Geometry: final body of the model. Coordinates: model frame, mm. Face numbers are marked on the shaded views. A direction names the side the tool comes from. Give positions to 0.01 mm unless a question says otherwise; leave off trailing zeros. Write each loop counter-clockwise with the first axis right and the second up, starting at its lowest first coordinate (ties: lowest second). Pieces come first, ordered by that corner, then holes. Notation, with made-up numbers: (-31.75, 80) -> (-19.75, 80) arc R18 cw to (-19.75, 94) -> close; hole circle Ø9 at (47.25, 84). An arc over 180 degrees is marked (long way). Answer in a Markdown table with one row per item. Add a question column.
Item 1: First-contact query: P1, Ø6.5, axis at x = 0, z = 0, coming from the -Y side; P2, Ø1.5, axis at y = 2.5, z = -1.5, coming from the +X side; P3, Ø2, axis at x = 4.5, y = 1.5, coming from the +Z side. Flat tips, straight axial feed; report the tip coordinate or a pass-through.
Item 2: Material intervals for probe 1 along Z at (x, y) = (0, 0.1); probe 2 along Z at (x, y) = (0, 3.95); probe 3 along X at (y, z) = (3.9, 0), sorted ascending. Write a range as from..to.
Item 3: Access query for the marked faces 1 and 2. Directions: +Z, -Z, +X, -X, +Y, -Y. A direction counts if a zero-diameter tool reaches every point of the face in a straight line with its end or side. Return the directions, or none.
Item 4: Section query C-C on y = 1.4. Output: boundary loops of the cut face in (x, z), plus the area to 3 significant figures.
Item 5: Draft query along Z for the marked faces 3, 4 and 5. Return one class per face: +Z half, -Z half, draft (parallel to the pull), parting line (faces both ways), or undercut.
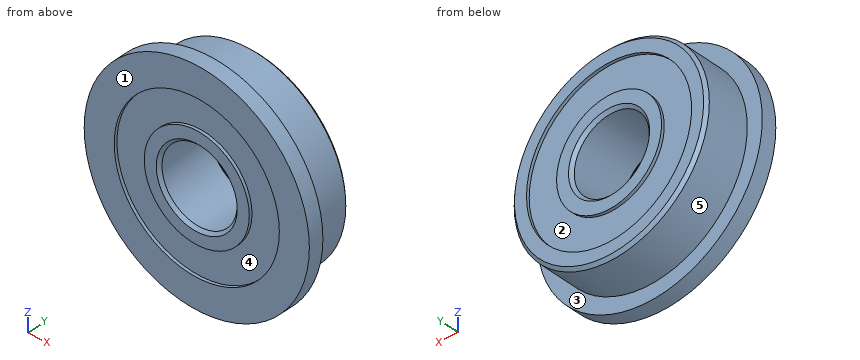
```python
from build123d import *

# Parameters (mm, degrees)
SKETCH3_R          = 5.5
SKETCH3_R_2        = 3.5
CUT_EXTRUDE1_DEPTH = 0.2
CHAMFER1_SIZE      = 0.2


with BuildPart() as part:
    # Sketch2 → Revolve1 (revolve)
    with BuildSketch(Plane.XY):
        Polygon((-6.5, 4), (-2.5, 4), (-2.5, 0), (-7.5, 0), (-7.5, 1), (-6.5, 1), align=None)
    revolve(axis=Axis((0, 1.921623867, 0), (0, -1, 0)))

    # Sketch3 → Cut-Extrude1 (cut)
    with BuildSketch(Plane(origin=(0, 4, 0), x_dir=(1, 0, 0), z_dir=(0, 1, 0))):
        Circle(SKETCH3_R)
        Circle(SKETCH3_R_2, mode=Mode.SUBTRACT)
    cut_extrude1 = extrude(amount=-CUT_EXTRUDE1_DEPTH, mode=Mode.SUBTRACT)

    # Mirror1: Cut-Extrude1 across plane
    add(cut_extrude1.mirror(Plane.ZX.offset(2)), mode=Mode.SUBTRACT)

    # Chamfer1
    chamfer1_edges = [part.edges().sort_by_distance(p)[0] for p in [
        (2.5, 0, 0),
        (2.5, 4, 0),
        (6.5, 4, 0),
    ]]
    chamfer(chamfer1_edges, length=CHAMFER1_SIZE)


solid = part.part
```
Findings below:
| question | item | result |
|---|---|---|
| 1 | P1 | stops at y = 0 |
| 1 | P2 | stops at x = 6.46 |
| 1 | P3 | stops at z = 6.56 |
| 2 | probe 1 | z = -7.5..-5.5, -3.5..-2.6, 2.6..3.5, 5.5..7.5 |
| 2 | probe 2 | z = -6.35..-5.5, -3.5..-2.65, 2.65..3.5, 5.5..6.35 |
| 2 | probe 3 | x = -6.4..-5.5, -3.5..-2.6, 2.6..3.5, 5.5..6.4 |
| 3 | face 1 | +Z, -Z, +X, -X, -Y |
| 3 | face 2 | +Y |
| 4 | outline | circle Ø13 at (0, 0); hole circle Ø5 at (0, 0) |
| 4 | area | 113 mm^2 |
| 5 | face 3 | draft |
| 5 | face 4 | undercut |
| 5 | face 5 | parting line |
